Geometry: final body of the model. Coordinates: model frame, mm. A direction names the side the tool comes from. Give positions to 0.01 mm unless a question says otherwise; leave off trailing zeros. Write each loop counter-clockwise with the first axis right and the second up, starting at its lowest first coordinate (ties: lowest second). Pieces come first, ordered by that corner, then holes. Notation, with made-up numbers: (47, -16) -> (74, -16) arc R23 cw to (74, 11) -> close; hole circle Ø7 at (22.5, 48). An arc over 180 degrees is marked (long way). Answer in a Markdown table with one row per item. Add a question column.
from build123d import *

# Parameters (mm, degrees)
SKETCH1_R               = 2.5
BOSS_EXTRUDE1_DEPTH     = 2
BOSS_EXTRUDE1_2_DEPTH   = 2
BOSS_EXTRUDE3_OUTLINE_R = 2.5
BOSS_EXTRUDE3_DEPTH     = 2
SKETCH6_R               = 5
CUT_EXTRUDE1_DEPTH      = 4
CUT_EXTRUDE2_START      = -10
CUT_EXTRUDE2_DEPTH      = 10
BOSS_EXTRUDE4_START     = 1
SKETCH8_R               = 7
SKETCH8_R_2             = 5
BOSS_EXTRUDE4_DEPTH     = 1


# Read off the part's stored shape, not the designer's step: Boss-Extrude3
with BuildPart() as part:
    # Sketch1 → Boss-Extrude1 (new body)
    with BuildSketch(Plane(origin=(0, 0, 0), x_dir=(1, 0, 0), z_dir=(0, 1, 0))):
        with BuildLine():
            ThreePointArc((23.674984177, 34.026642345), (27.138423224, 37.66837111), (31.041417883, 40.83447773))
            Line((31.041417883, 40.83447773), (24.387097577, 50.213711241))
            ThreePointArc((24.387097577, 50.213711241), (20.045094669, 46.759453741), (16.108243271, 42.849711395))
            ThreePointArc((16.108243271, 42.849711395), (12.171391874, 46.759453741), (7.829388966, 50.213711241))
            Line((7.829388966, 50.213711241), (1.175068659, 40.83447773))
            ThreePointArc((1.175068659, 40.83447773), (5.078063318, 37.66837111), (8.541502365, 34.026642345))
            Line((8.541502365, 34.026642345), (23.674984177, 34.026642345))
        make_face()
        with Locations(Location((11.108243271, 39.026642345, 0), (0, 0, 270))):
            Circle(SKETCH1_R, mode=Mode.SUBTRACT)
        with Locations(Location((21.108243271, 39.026642345, 0), (0, 0, 270))):
            Circle(SKETCH1_R, mode=Mode.SUBTRACT)
    extrude(amount=BOSS_EXTRUDE1_DEPTH)



with BuildPart() as body_2:
    # Sketch1 → Boss-Extrude1 2 (new body)
    with BuildSketch(Plane(origin=(0, 0, 0), x_dir=(1, 0, 0), z_dir=(0, 1, 0))):
        with BuildLine():
            Line((24.387097577, -32.160426552), (31.041417883, -22.781193041))
            ThreePointArc((31.041417883, -22.781193041), (27.138423224, -19.615086421), (23.674984177, -15.973357655))
            Line((23.674984177, -15.973357655), (8.541502365, -15.973357655))
            ThreePointArc((8.541502365, -15.973357655), (5.078063318, -19.615086421), (1.175068659, -22.781193041))
            Line((1.175068659, -22.781193041), (7.829388966, -32.160426552))
            ThreePointArc((7.829388966, -32.160426552), (12.171391874, -28.706169052), (16.108243271, -24.796426706))
            ThreePointArc((16.108243271, -24.796426706), (20.045094669, -28.706169052), (24.387097577, -32.160426552))
        make_face()
        with Locations(Location((11.108243271, -20.973357655, 0), (0, 0, 270))):
            Circle(SKETCH1_R, mode=Mode.SUBTRACT)
        with Locations(Location((21.108243271, -20.973357655, 0), (0, 0, 270))):
            Circle(SKETCH1_R, mode=Mode.SUBTRACT)
    extrude(amount=BOSS_EXTRUDE1_2_DEPTH)


with BuildPart() as part_1:
    add(part.part)

    add(body_2.part)  # Boss-Extrude3 merges body 2
    # Boss-Extrude3 outline → Boss-Extrude3 (add)
    with BuildSketch(Plane(origin=(0, 2, 0), x_dir=(1, 0, 0), z_dir=(0, 1, 0))):
        with BuildLine():
            ThreePointArc((16.108243271, 42.849711395), (12.171391874, 46.759453741), (7.829388966, 50.213711241))
            Line((7.829388966, 50.213711241), (1.175068659, 40.83447773))
            ThreePointArc((1.175068659, 40.83447773), (5.078063318, 37.66837111), (8.541502365, 34.026642345))
            Line((8.541502365, 34.026642345), (8.541502365, -15.973357655))
            ThreePointArc((8.541502365, -15.973357655), (5.078063318, -19.615086421), (1.175068659, -22.781193041))
            Line((1.175068659, -22.781193041), (7.829388966, -32.160426552))
            ThreePointArc((7.829388966, -32.160426552), (12.171391874, -28.706169052), (16.108243271, -24.796426706))
            ThreePointArc((16.108243271, -24.796426706), (20.045094669, -28.706169052), (24.387097577, -32.160426552))
            Line((24.387097577, -32.160426552), (31.041417883, -22.781193041))
            ThreePointArc((31.041417883, -22.781193041), (27.138423224, -19.615086421), (23.674984177, -15.973357655))
            Line((23.674984177, -15.973357655), (23.674984177, 34.026642345))
            ThreePointArc((23.674984177, 34.026642345), (27.138423224, 37.66837111), (31.041417883, 40.83447773))
            Line((31.041417883, 40.83447773), (24.387097577, 50.213711241))
            ThreePointArc((24.387097577, 50.213711241), (20.045094669, 46.759453741), (16.108243271, 42.849711395))
        make_face()
        with Locations((11.108243271, -20.973357655)):
            Circle(BOSS_EXTRUDE3_OUTLINE_R, mode=Mode.SUBTRACT)
        with Locations((21.108243271, -20.973357655)):
            Circle(BOSS_EXTRUDE3_OUTLINE_R, mode=Mode.SUBTRACT)
        with Locations((11.108243271, 39.026642345)):
            Circle(BOSS_EXTRUDE3_OUTLINE_R, mode=Mode.SUBTRACT)
        with Locations((21.108243271, 39.026642345)):
            Circle(BOSS_EXTRUDE3_OUTLINE_R, mode=Mode.SUBTRACT)
    extrude(amount=BOSS_EXTRUDE3_DEPTH)

    # Sketch6 → Cut-Extrude1 (cut)
    with BuildSketch(Plane(origin=(0, 4, 0), x_dir=(1, 0, 0), z_dir=(0, 1, 0))):
        with Locations(Location((16.108243271, 9.024711395, 0), (0, 0, 270))):
            Circle(SKETCH6_R)
    extrude(amount=-CUT_EXTRUDE1_DEPTH, mode=Mode.SUBTRACT)

    # Sketch7 → Cut-Extrude2 (cut)
    with BuildSketch(Plane(origin=(0, 4, 0), x_dir=(1, 0, 0), z_dir=(0, 1, 0)).offset(CUT_EXTRUDE2_START)):
        with BuildLine():
            Line((1.175068659, -22.781193041), (7.829388966, -32.160426552))
            ThreePointArc((7.829388966, -32.160426552), (12.171391874, -28.706169052), (16.108243271, -24.796426706))
            ThreePointArc((16.108243271, -24.796426706), (20.045094669, -28.706169052), (24.387097577, -32.160426552))
            Line((24.387097577, -32.160426552), (31.041417883, -22.781193041))
            ThreePointArc((31.041417883, -22.781193041), (27.138423224, -19.615086421), (23.674984177, -15.973357655))
            Line((23.674984177, -15.973357655), (23.674984177, 34.026642345))
            ThreePointArc((23.674984177, 34.026642345), (27.138423224, 37.66837111), (31.041417883, 40.83447773))
            Line((31.041417883, 40.83447773), (24.387097577, 50.213711241))
            ThreePointArc((24.387097577, 50.213711241), (20.045094669, 46.759453741), (16.108243271, 42.849711395))
            ThreePointArc((16.108243271, 42.849711395), (12.171391874, 46.759453741), (7.829388966, 50.213711241))
            Line((7.829388966, 50.213711241), (1.175068659, 40.83447773))
            ThreePointArc((1.175068659, 40.83447773), (5.078063318, 37.66837111), (8.541502365, 34.026642345))
            Line((8.541502365, 34.026642345), (8.541502365, -15.973357655))
            ThreePointArc((8.541502365, -15.973357655), (5.078063318, -19.615086421), (1.175068659, -22.781193041))
        make_face()
        with BuildLine():
            Line((1.870348493, -22.897086458), (7.946416825, -31.461276502))
            ThreePointArc((7.946416825, -31.461276502), (12.232412061, -27.97896903), (16.108243271, -24.045249044))
            ThreePointArc((16.108243271, -24.045249044), (19.984074481, -27.97896903), (24.270069717, -31.461276502))
            Line((24.270069717, -31.461276502), (30.34613805, -22.897086458))
            ThreePointArc((30.34613805, -22.897086458), (26.549691802, -19.749820127), (23.174984177, -16.154039555))
            Line((23.174984177, -16.154039555), (23.174984177, 34.207324244))
            ThreePointArc((23.174984177, 34.207324244), (26.549691802, 37.803104816), (30.34613805, 40.950371147))
            Line((30.34613805, 40.950371147), (24.270069717, 49.514561191))
            ThreePointArc((24.270069717, 49.514561191), (19.984074481, 46.032253719), (16.108243271, 42.098533733))
            ThreePointArc((16.108243271, 42.098533733), (12.232412061, 46.032253719), (7.946416825, 49.514561191))
            Line((7.946416825, 49.514561191), (1.870348493, 40.950371147))
            ThreePointArc((1.870348493, 40.950371147), (5.666794741, 37.803104816), (9.041502365, 34.207324244))
            Line((9.041502365, 34.207324244), (9.041502365, -16.154039555))
            ThreePointArc((9.041502365, -16.154039555), (5.666794741, -19.749820127), (1.870348493, -22.897086458))
        make_face(mode=Mode.SUBTRACT)
    extrude(amount=CUT_EXTRUDE2_DEPTH, mode=Mode.SUBTRACT)

    # Sketch8 → Boss-Extrude4 (add)
    with BuildSketch(Plane(origin=(0, 4, 0), x_dir=(1, 0, 0), z_dir=(0, 1, 0)).offset(BOSS_EXTRUDE4_START)):
        with Locations(Location((16.108243271, 9.024711395, 0), (0, 0, 270))):
            Circle(SKETCH8_R)
        with Locations(Location((16.108243271, 9.024711395, 0), (0, 0, 270))):
            Circle(SKETCH8_R_2, mode=Mode.SUBTRACT)
    extrude(amount=-BOSS_EXTRUDE4_DEPTH)


solid = part_1.part
Q1. Section B-B on z = -9. Return loops of the section in (x, y), and give its area (3 significant figures).
Q2. Access query for faces 4 (the cylindrical face through (12.29, 1.97, -45.98)), 5 (the cylindrical face through (5.616, 1.972, -37.85)), 6 (the flat face through (16, 1, -34.027)). Directions: +Z, -Z, +X, -X, +Y, -Y. A direction counts if a zero-diameter tool reaches every point of the face in a straight line with its end or side. Return the directions, or none.
Q3. Pull-direction query (Z, two-part tool) for faces 1 (the flat face through (16, 4, -1)), 2 (the flat face through (23.175, 3, -9)), 3 (the flat face through (4.95, 1.97, -45.29)); classes: +Z half, -Z half, draft (parallel to the pull), parting line (faces both ways), or undercut.
Q4. Section C-C on y = 3.05. Return loops of the section in (x, z), and give its area (3 significant figures).
Q5. Line query: probe 1 along Z at (x, y) = (9.25, 0.9); probe 2 along Z at (x, y) = (12, 3.35); probe 3 along X at (y, z) = (1.95, 20). Output: solid intervals per line, ascending. Write a range as from..to.
Q6. Contact query for flat-ended pins moving along their axis: pin 1 Ø2 at (y, z) = (2, 6) entering from +X (3 decimals); pin 2 Ø8.5 at (x, z) = (10, -13.5) entering from +Y; pin 3 Ø2 at (x, y) = (12.5, 0.5) entering from -Z; pin 4 Ø3 at (y, z) = (3, -7) entering from -X. Output: stop coordinate, or through.
Q7. Section A-A on x = 14.5. Return loops of the section in (y, z).
Q8. Section D-D on x = 27.25. Return loops of the section in (y, z).
Checks:
| question | item | result |
|---|---|---|
| 1 | outline | (9.04, 2) -> (11.11, 2) -> (11.11, 5) -> (9.11, 5) -> (9.11, 4) -> (9.04, 4) -> close; (21.11, 2) -> (23.17, 2) -> (23.17, 4) -> (23.11, 4) -> (23.11, 5) -> (21.11, 5) -> close |
| 1 | area | 12.3 mm^2 |
| 2 | face 4 | -Z, +Y, -Y |
| 2 | face 5 | -X, +Y, -Y |
| 2 | face 6 | +X, -X, -Y |
| 3 | face 1 | draft |
| 3 | face 2 | undercut |
| 3 | face 3 | -Z half |
| 4 | outline | (1.87, -40.95) -> (7.95, -49.51) arc R50 ccw to (16.11, -42.1) arc R50 ccw to (24.27, -49.51) -> (30.35, -40.95) arc R39.5 cw to (23.17, -34.21) -> (23.17, 16.15) arc R39.5 cw to (30.35, 22.9) -> (24.27, 31.46) arc R50 ccw to (16.11, 24.05) arc R50 ccw to (7.95, 31.46) -> (1.87, 22.9) arc R39.5 cw to (9.04, 16.15) -> (9.04, -34.21) arc R39.5 cw to start; hole circle Ø5 at (11.11, -39.03); hole circle Ø5 at (11.11, 20.97); hole circle Ø10 at (16.11, -9.02); hole circle Ø5 at (21.11, -39.03); hole circle Ø5 at (21.11, 20.97) |
| 4 | area | 1,110 mm^2 |
| 5 | probe 1 | -48.54..-40.7, -37.35..-34.03, 15.97..19.3, 22.65..30.48 |
| 5 | probe 2 | -46.24..-41.36, -36.69..-11.87, -6.17..18.64, 23.31..28.19 |
| 5 | probe 3 | 5.4..8.81, 13.41..18.81, 23.41..26.82 |
| 6 | pin 1 | x = 23.175 |
| 6 | pin 2 | y = 5 |
| 6 | pin 3 | z = -46.68 |
| 6 | pin 4 | x = 9.04 |
| 7 | outline | (0, -43.84) -> (4, -43.84) -> (4, -15.84) -> (5, -15.84) -> (5, -13.76) -> (2, -13.76) -> (2, -34.03) -> (0, -34.03) -> close; (0, 15.97) -> (2, 15.97) -> (2, -4.29) -> (5, -4.29) -> (5, -2.21) -> (4, -2.21) -> (4, 25.78) -> (0, 25.78) -> close |
| 8 | outline | (0, -45.31) -> (4, -45.31) -> (4, -38.45) -> (0, -38.45) -> close; (0, 20.39) -> (4, 20.39) -> (4, 27.26) -> (0, 27.26) -> close |
